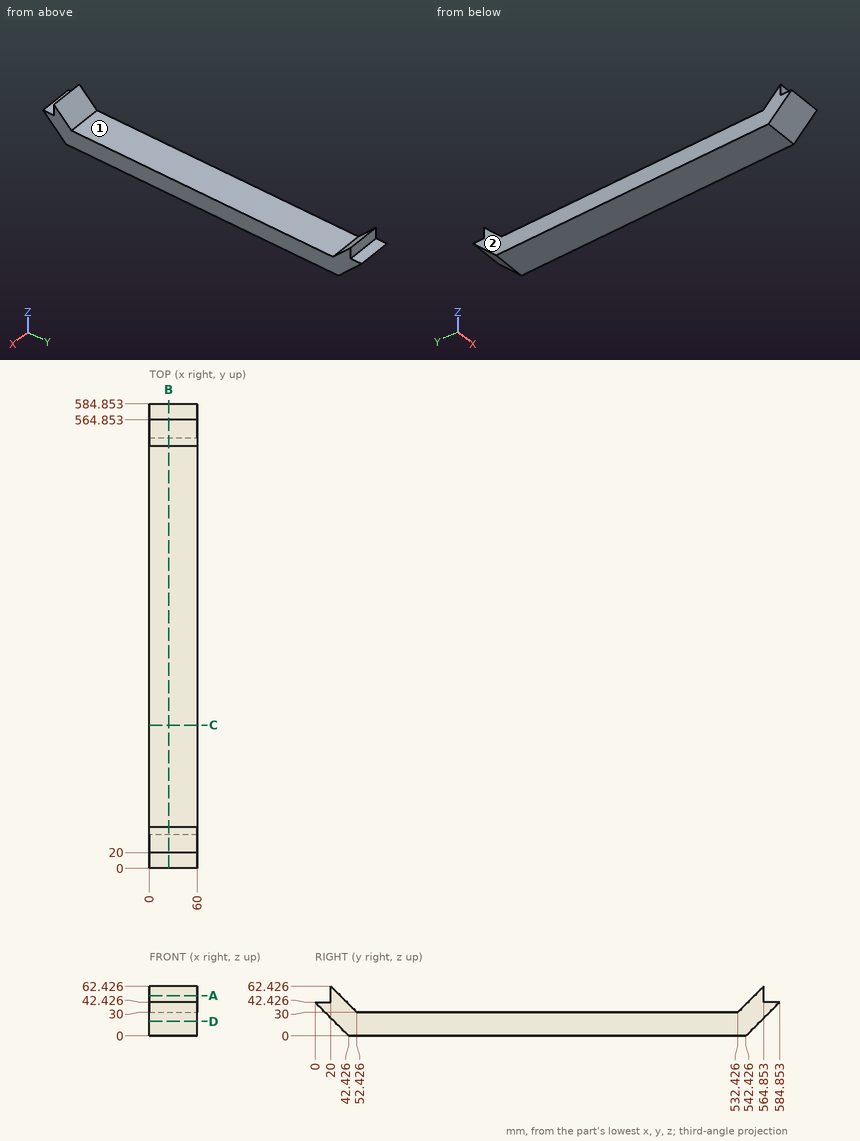
The drawing under review shows one solid part. Ordinate dimensions are in mm from its lowest x, y, z. A direction names the side the tool comes from. Round coordinates to 2 decimals unless told otherwise and drop trailing zeros. Write each loop counter-clockwise with the first axis right and the second up, starting at its lowest first coordinate (ties: lowest second). Pieces come first, ordered by that corner, then holes. Notation, with made-up numbers: M 54,-28 L 77,-28 A15 cw 77,-21 Z; hole C 41,-4 d5. An arc over 180 degrees is marked long. One line per item, written item: value. Start each with the question number.
(1) We need section A-A (z = 51). Give the boundary of the cut face in (x, y).
(2) Insertion check: pin 1 (16 mm diameter, centred on x = 29, y = 11, fed in from +Z); pin 2 (6 mm diameter, centred on x = 26, z = 52.5, fed in from +Y); pin 3 (5 mm diameter, centred on x = 42.5, z = 19.5, fed in from -Y) (1 decimal). Each pin has a flat end and moves straight along its axis. Give the tip position at first contact, or say it passes through.
(3) We need section C-C (y = 180.5). Give the boundary of the cut face in (x, z), and give its area (3 significant figures).
(4) We need section B-B (x = 24). Give the boundary of the cut face in (y, z).
(5) We need section D-D (z = 18.5). Give the boundary of the cut face in (x, y), and give its area (3 significant figures).
(6) Wall thickness on line 1 (Z direction, x = 37.5, y = 496); line 2 (Y direction, x = 16.5, z = 60) (1 decimal); line 3 (Y direction, x = 35, z = 53) (1 decimal): over which ranges is each line inside the solid? List them lowest first.
(7) Machinability: for the marked faces 1 and 2, which of the approach directions +Z, -Z, +X, -X, +Y, -Y give a long, thin tool a straight path to every point of the face, cutting with its end or side? Answer none if there is none.
Result:
1. outline: M 0,20 L 60,20 L 60,31.43 L 0,31.43 Z; M 0,553.43 L 60,553.43 L 60,564.85 L 0,564.85 Z
2. pin 1: z = 42.43
2. pin 2: y = 564.85
2. pin 3: y = 20.4
3. outline: M 0,0 L 60,0 L 60,30 L 0,30 Z
3. area: 1,800 mm²
4. outline: M 0,42.43 L 42.43,0 L 542.43,0 L 584.85,42.43 L 564.85,42.43 L 564.85,62.43 L 532.43,30 L 52.43,30 L 20,62.43 L 20,42.43 Z
5. outline: M 0,23.93 L 60,23.93 L 60,560.93 L 0,560.93 Z
5. area: 32,200 mm²
6. line 1: 0 to 30
6. line 2: 20 to 22.4, 562.4 to 564.9
6. line 3: 20 to 29.4, 555.4 to 564.9
7. face 1: +Z, +X, -X
7. face 2: +Z, -Z, -X, +Y, -Y
